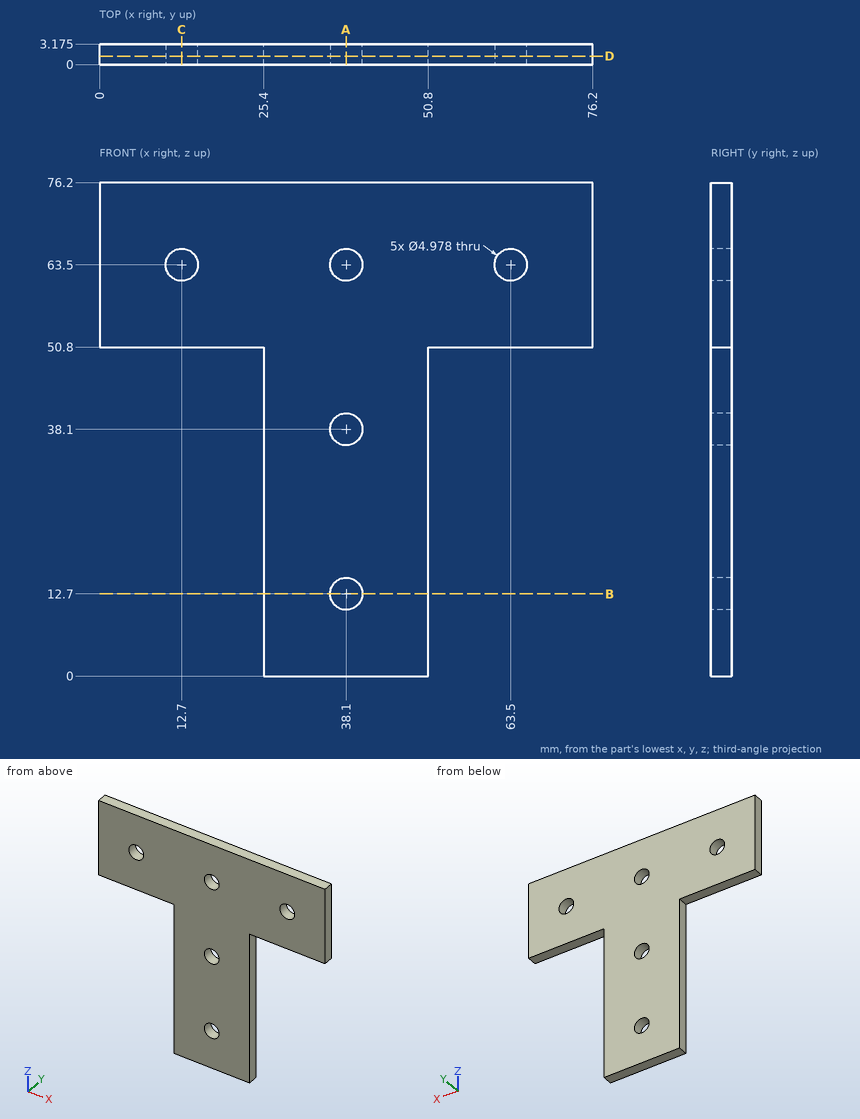
Answer from the drawing. Dimensions are ordinates in mm from the lowest x, y and z of the part. Coordinates: 2 decimals unless noted, no trailing zeros. Write each loop counter-clockwise with the first axis right and the second up, starting at its lowest first coordinate (ties: lowest second). Pieces come first, ordered by that corner, then holes. Notation, with made-up numbers: M -36.5,-24.5 L -18.5,-24.5 A28 cw -18.5,13.5 Z; hole C 88,-31 d11. An arc over 180 degrees is marked long. Put each result on its own line as item: value. Start each with the question number.
1. A cutting plane is placed at B-B on z = 12.7. Write down the section's boundary in (x, y) (1 decimal).
2. A cutting plane is placed at C-C on x = 12.7. Write down the section's boundary in (y, z) (1 decimal).
3. A cutting plane is placed at A-A on x = 38.1. Write down the section's boundary in (y, z) (1 decimal).
4. Flat-ended cylindrical pins translate along their axes: P1, Ø4.5, axis at x = 12.7, z = 63.5, coming from the -Y side; P2, Ø1, axis at x = 16, y = 1.5, coming from the -Z side; P3, Ø1, axis at y = 1.5, z = 26, coming from the -X side. Find the tip coordinate at first contact, or state that the pin passes through.
5. Consider line 1 (Z direction, x = 38.1, y = 1.35); line 2 (X direction, y = 0.75, z = 38.1). Determine where each line is inside the solid, lowest interval first. Write a range as from..to.
6. A cutting plane is placed at D-D on y = 1.3. Write down the section's boundary in (x, z).
Resolved:
1. outline: M 25.4,0 L 35.6,0 L 35.6,3.2 L 25.4,3.2 Z; M 40.6,0 L 50.8,0 L 50.8,3.2 L 40.6,3.2 Z
2. outline: M 0,50.8 L 3.2,50.8 L 3.2,61 L 0,61 Z; M 0,66 L 3.2,66 L 3.2,76.2 L 0,76.2 Z
3. outline: M 0,0 L 3.2,0 L 3.2,10.2 L 0,10.2 Z; M 0,15.2 L 3.2,15.2 L 3.2,35.6 L 0,35.6 Z; M 0,40.6 L 3.2,40.6 L 3.2,61 L 0,61 Z; M 0,66 L 3.2,66 L 3.2,76.2 L 0,76.2 Z
4. P1: passes through
4. P2: stops at z = 50.8
4. P3: stops at x = 25.4
5. line 1: z = 0..10.21, 15.19..35.61, 40.59..61.01, 65.99..76.2
5. line 2: x = 25.4..35.61, 40.59..50.8
6. outline: M 0,50.8 L 25.4,50.8 L 25.4,0 L 50.8,0 L 50.8,50.8 L 76.2,50.8 L 76.2,76.2 L 0,76.2 Z; hole C 12.7,63.5 d4.98; hole C 38.1,12.7 d4.98; hole C 38.1,38.1 d4.98; hole C 38.1,63.5 d4.98; hole C 63.5,63.5 d4.98
